Input: part model. Units: mm. Frame: model coordinates. Face numbers are marked on the shaded views. Give positions to 0.01 mm unless a question says otherwise; leave off trailing zeros. Loops run counter-clockwise (first coordinate to the right, second up) from the corner with the lowest first, then second, coordinate; pieces in that order, holes last. Notation, with made-up numbers: M 45,6.5 L 93,6.5 A23 cw 93,29.5 Z; hole C 50,15.25 d2. An arc over 180 degrees is marked long. Return JSON: item names as keys, results as strings. Group by question number.
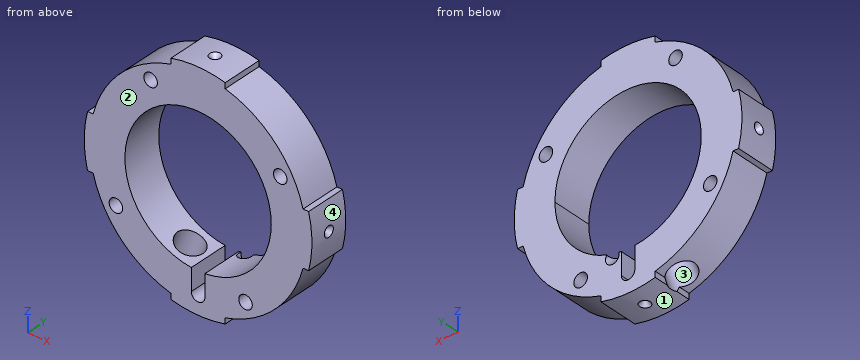
```python
from build123d import *

# Parameters (mm, degrees)
SKETCH1_R               = 40
BOSS_EXTRUDE1_DEPTH     = 15
BOSS_EXTRUDE2_DEPTH     = 15
CIRPATTERN1_COUNT       = 4
CUT_EXTRUDE1_REACH      = 102.194
CUT_EXTRUDE1_END_RADIUS = 27
SKETCH3_R               = 5
CUT_EXTRUDE2_REACH      = 63.262
SKETCH7_R               = 2.5
CIRPATTERN2_COUNT       = 4


with BuildPart() as part:
    # Sketch1 → Boss-Extrude1 (new body)
    with BuildSketch(Plane(origin=(0, 0, 0), x_dir=(1, 0, 0), z_dir=(0, 1, 0))):
        with Locations(Location((0, 0, 0), (0, 0, 270))):
            Circle(SKETCH1_R)
        with BuildLine():
            Line((-2.5, 26.884010118), (-2.5, 35))
            ThreePointArc((-2.5, 35), (0, 37.5), (2.5, 35))
            Line((2.5, 35), (2.5, 26.884010118))
            ThreePointArc((2.5, 26.884010118), (19.956202043, 18.186533479), (27, 0))
            ThreePointArc((27, 0), (-18.186533479, -19.956202043), (-2.5, 26.884010118))
        make_face(mode=Mode.SUBTRACT)
    extrude(amount=BOSS_EXTRUDE1_DEPTH)

    # Sketch2 → Boss-Extrude2 (add)
    with BuildSketch(Plane(origin=(0, 0, 0), x_dir=(1, 0, 0), z_dir=(0, 1, 0))):
        with BuildLine():
            Line((-10, 38.729833462), (-10, 40.792156109))
            ThreePointArc((-10, 40.792156109), (0, 42), (10, 40.792156109))
            Line((10, 40.792156109), (10, 38.729833462))
            ThreePointArc((10, 38.729833462), (0, 40), (-10, 38.729833462))
        make_face()
    boss_extrude2 = extrude(amount=BOSS_EXTRUDE2_DEPTH)

    # CirPattern1: Boss-Extrude2 ×4 about axis
    cirpattern1_axis = Axis((0, 0, 0), (0, 1, 0))
    for i in range(1, CIRPATTERN1_COUNT):
        add(boss_extrude2.rotate(cirpattern1_axis, i * 360 / CIRPATTERN1_COUNT))

    # Cut-Extrude1: up to this cylinder (the profile starts outside it)
    cut_extrude1_end = Plane(origin=(0, 7.5, 0), z_dir=(0, -1, 0)) * Cylinder(CUT_EXTRUDE1_END_RADIUS, 259.388, mode=Mode.PRIVATE)
    # Sketch3 → Cut-Extrude1 (cut, up to the surface)
    with BuildSketch(Plane(origin=(-14.36484602, 0, -39.467090073), x_dir=(0, -1, 0), z_dir=(-0.34202014332566616, 0, -0.9396926207859094)), mode=Mode.PRIVATE) as cut_extrude1_sk1:
        with Locations(Location((-7.5, 0, 0), (0, 0, 90))):
            Circle(SKETCH3_R)
    cut_extrude1_tool1 = extrude(cut_extrude1_sk1.sketch, amount=-CUT_EXTRUDE1_REACH, mode=Mode.PRIVATE) - cut_extrude1_end
    add(cut_extrude1_tool1.solids().sort_by_distance((-14.364846, 7.5, -39.46709))[0], mode=Mode.SUBTRACT)

    # Cut-Loft1: read off the stored shape, not the designer's step
    # Cut-Loft1: loft between two sections, ruled curve by curve
    cut_loft1_from = [
        Edge.make_bspline([(3.514240275, 15, -26.425622361), (3.43403107, 15, -26.617896283), (3.366678926, 15, -26.845149984), (3.307378731, 15, -27.375176333), (3.316276229, 15, -27.679385236), (3.439149004, 15, -28.164052423), (3.499144635, 15, -28.33030076), (3.660731431, 15, -28.657904123), (3.762322597, 15, -28.819259148), (4.01061992, 15, -29.122797357), (4.156634299, 15, -29.264354751), (4.484735709, 15, -29.510646827), (4.666742961, 15, -29.615210684), (5.051290806, 15, -29.775629094), (5.253649364, 15, -29.831407709), (5.659510988, 15, -29.891296475), (5.862836528, 15, -29.895470114), (6.253234588, 15, -29.858370786), (6.439375692, 15, -29.817046477), (6.785871072, 15, -29.701395244), (6.946225348, 15, -29.627068321), (7.37710147, 15, -29.373403645), (7.599547955, 15, -29.165702458), (7.934492045, 15, -28.750664024), (8.048605206, 15, -28.542917202), (8.209023616, 15, -28.158369358), (8.27637576, 15, -27.931115657), (8.335675954, 15, -27.401089308), (8.326778456, 15, -27.096880405), (8.203905682, 15, -26.612213219), (8.143910051, 15, -26.445964881), (7.982323255, 15, -26.118361518), (7.880732089, 15, -25.957006493), (7.632434766, 15, -25.653468284), (7.486420387, 15, -25.51191089), (7.158318977, 15, -25.265618814), (6.976311725, 15, -25.161054957), (6.59176388, 15, -25.000636547), (6.389405322, 15, -24.944857932), (5.983543698, 15, -24.884969166), (5.780218158, 15, -24.880795527), (5.389820098, 15, -24.917894855), (5.203678994, 15, -24.959219164), (4.857183614, 15, -25.074870397), (4.696829338, 15, -25.14919732), (4.265953216, 15, -25.402861996), (4.043506731, 15, -25.610563184), (3.708562641, 15, -26.025601617), (3.59444948, 15, -26.233348439), (3.514240275, 15, -26.425622361)], [0, 0, 0, 0, 0.0625, 0.0625, 0.125, 0.125, 0.15625, 0.15625, 0.1875, 0.1875, 0.21875, 0.21875, 0.25, 0.25, 0.28125, 0.28125, 0.3125, 0.3125, 0.34375, 0.34375, 0.375, 0.375, 0.4375, 0.4375, 0.5, 0.5, 0.5625, 0.5625, 0.625, 0.625, 0.65625, 0.65625, 0.6875, 0.6875, 0.71875, 0.71875, 0.75, 0.75, 0.78125, 0.78125, 0.8125, 0.8125, 0.84375, 0.84375, 0.875, 0.875, 0.9375, 0.9375, 1, 1, 1, 1], 3),
    ]
    cut_loft1_to = [
        Edge.make_bspline([(2.074985381, 12, -24.185039409), (2.13411013, 12, -24.427947342), (2.230529651, 12, -24.695535226), (2.549951041, 12, -25.250125143), (2.77479132, 12, -25.537914734), (3.238098263, 12, -25.919158327), (3.413256539, 12, -26.037240227), (3.802322838, 12, -26.239189581), (4.016282358, 12, -26.322904324), (4.47210154, 12, -26.439875089), (4.713892566, 12, -26.472945015), (5.206175894, 12, -26.477842878), (5.456469637, 12, -26.449562366), (5.942285504, 12, -26.331312867), (6.177577655, 12, -26.241399857), (6.612541462, 12, -26.010806383), (6.812086613, 12, -25.870313491), (7.163158835, 12, -25.556942174), (7.314710473, 12, -25.384260574), (7.567442578, 12, -25.026094956), (7.668738965, 12, -24.840722901), (7.90500687, 12, -24.28920003), (7.972433417, 12, -23.93027154), (8.001244839, 12, -23.290920383), (7.963900528, 12, -23.00895336), (7.845651029, 12, -22.523137493), (7.749231508, 12, -22.255549609), (7.429810118, 12, -21.700959692), (7.204969839, 12, -21.413170101), (6.741662897, 12, -21.031926508), (6.56650462, 12, -20.913844608), (6.177438321, 12, -20.711895254), (5.963478802, 12, -20.628180512), (5.507659619, 12, -20.511209746), (5.265868593, 12, -20.47813982), (4.773585266, 12, -20.473241957), (4.523291522, 12, -20.50152247), (4.037475655, 12, -20.619771968), (3.802183505, 12, -20.709684978), (3.367219697, 12, -20.940278452), (3.167674546, 12, -21.080771344), (2.816602324, 12, -21.394142661), (2.665050687, 12, -21.566824261), (2.412318581, 12, -21.924989879), (2.311022194, 12, -22.110361934), (2.074754289, 12, -22.661884805), (2.007327743, 12, -23.020813295), (1.97851632, 12, -23.660164452), (2.015860632, 12, -23.942131475), (2.074985381, 12, -24.185039409)], [0, 0, 0, 0, 0.0625, 0.0625, 0.125, 0.125, 0.15625, 0.15625, 0.1875, 0.1875, 0.21875, 0.21875, 0.25, 0.25, 0.28125, 0.28125, 0.3125, 0.3125, 0.34375, 0.34375, 0.375, 0.375, 0.4375, 0.4375, 0.5, 0.5, 0.5625, 0.5625, 0.625, 0.625, 0.65625, 0.65625, 0.6875, 0.6875, 0.71875, 0.71875, 0.75, 0.75, 0.78125, 0.78125, 0.8125, 0.8125, 0.84375, 0.84375, 0.875, 0.875, 0.9375, 0.9375, 1, 1, 1, 1], 3),
    ]
    cut_loft1 = Solid(Shell([*[Face.make_surface_from_curves(cut_loft1_from[k], cut_loft1_to[k]) for k in range(1)], Face(Wire(cut_loft1_from)), Face(Wire(cut_loft1_to))]))
    add(cut_loft1, mode=Mode.SUBTRACT)

    # Sketch7 → Cut-Extrude2 (cut, up to next)
    with BuildSketch(Plane(origin=(0, 15, 0), x_dir=(1, 0, 0), z_dir=(0, 1, 0)), mode=Mode.PRIVATE) as cut_extrude2_sk1:
        with Locations(Location((17.5, 30.310889132, 0), (0, 0, 270))):
            Circle(SKETCH7_R)
    cut_extrude2_tool1 = extrude(cut_extrude2_sk1.sketch, amount=-CUT_EXTRUDE2_REACH, mode=Mode.PRIVATE) & part.part
    # Sketch7 → Cut-Extrude2 (cut, up to next)
    with BuildSketch(Plane(origin=(0, 15, 0), x_dir=(1, 0, 0), z_dir=(0, 1, 0)), mode=Mode.PRIVATE) as cut_extrude2_sk2:
        with Locations(Location((30.310889132, -17.5, 0), (0, 0, 270))):
            Circle(SKETCH7_R)
    cut_extrude2_tool2 = extrude(cut_extrude2_sk2.sketch, amount=-CUT_EXTRUDE2_REACH, mode=Mode.PRIVATE) & part.part
    # Sketch7 → Cut-Extrude2 (cut, up to next)
    with BuildSketch(Plane(origin=(0, 15, 0), x_dir=(1, 0, 0), z_dir=(0, 1, 0)), mode=Mode.PRIVATE) as cut_extrude2_sk3:
        with Locations(Location((-17.5, -30.310889132, 0), (0, 0, 270))):
            Circle(SKETCH7_R)
    cut_extrude2_tool3 = extrude(cut_extrude2_sk3.sketch, amount=-CUT_EXTRUDE2_REACH, mode=Mode.PRIVATE) & part.part
    # Sketch7 → Cut-Extrude2 (cut, up to next)
    with BuildSketch(Plane(origin=(0, 15, 0), x_dir=(1, 0, 0), z_dir=(0, 1, 0)), mode=Mode.PRIVATE) as cut_extrude2_sk4:
        with Locations(Location((-30.310889132, 17.5, 0), (0, 0, 270))):
            Circle(SKETCH7_R)
    cut_extrude2_tool4 = extrude(cut_extrude2_sk4.sketch, amount=-CUT_EXTRUDE2_REACH, mode=Mode.PRIVATE) & part.part
    add(cut_extrude2_tool1.solids().sort_by_distance((17.5, 15, -30.310889))[0], mode=Mode.SUBTRACT)
    add(cut_extrude2_tool2.solids().sort_by_distance((30.310889, 15, 17.5))[0], mode=Mode.SUBTRACT)
    add(cut_extrude2_tool3.solids().sort_by_distance((-17.5, 15, 30.310889))[0], mode=Mode.SUBTRACT)
    add(cut_extrude2_tool4.solids().sort_by_distance((-30.310889, 15, -17.5))[0], mode=Mode.SUBTRACT)

    # Sketch9 → Cut-Revolve4 (revolve, cut)
    with BuildSketch(Plane(origin=(0, 0, 0), x_dir=(0, 0, -1), z_dir=(1, 0, 0)), mode=Mode.PRIVATE) as cut_revolve4_sk:
        Polygon((42, 7.5), (42, 5.5), (40, 7.5), align=None)
    cut_revolve4 = revolve(cut_revolve4_sk.sketch.rotate(Axis((0, 7.5, -40), (0, 0, -1)), 180), axis=Axis((0, 7.5, -40), (0, 0, -1)), mode=Mode.SUBTRACT)

    # CirPattern2: Cut-Revolve4 ×4 about axis
    cirpattern2_axis = Axis((0, 15, 0), (0, -1, 0))
    for i in range(1, CIRPATTERN2_COUNT):
        add(cut_revolve4.rotate(cirpattern2_axis, i * 360 / CIRPATTERN2_COUNT), mode=Mode.SUBTRACT)


solid = part.part
```
Item 1: Section B-B, the plane z = 4. Return loops of the section in (x, y), then the cut area to 3 significant figures.
Item 2: Section C-C, the plane z = 17. Return loops of the section in (x, y).
Item 3: Pull-direction query (X, two-part tool) for the marked faces 1, 2, 3 and 4; classes: pulls with the +X half, pulls with the -X half, needs draft (parallel to the pull), parting line crosses it, or undercut.
Item 4: Material intervals for line 1 (X direction, y = 7.5, z = -17.5); line 2 (X direction, y = 4.75, z = 15.5); line 3 (X direction, y = 10.25, z = 0), sorted ascending. Write a range as from..to.
Item 5: First-contact query: pin 1 Ø0.6 at (x, y) = (-39.5, 7) entering from -Z; pin 2 Ø2 at (x, y) = (14, 3.5) entering from -Z; pin 3 Ø1 at (y, z) = (13, -39.5) entering from -X; pin 4 Ø6 at (x, z) = (-27, 32.5) entering from -Y. Flat tips, straight axial feed; report the tip coordinate or a pass-through.
Item 6: Section A-A, the plane z = -17.5. Return loops of the section in (x, y), then the cut area to 3 significant figures.
Answer below:
{
 "1": {"outline": "M -41.81,0 L -26.7,0 L -26.7,15 L -41.81,15 Z; M 26.7,0 L 41.81,0 L 41.81,15 L 26.7,15 Z", "area": "453 mm^2"},
 "2": {"outline": "M -36.21,0 L -20.98,0 L -20.98,15 L -36.21,15 Z; M 20.98,0 L 27.86,0 L 27.86,15 L 20.98,15 Z; M 32.76,0 L 36.21,0 L 36.21,15 L 32.76,15 Z"},
 "3": {"face 1": "parting line crosses it", "face 2": "needs draft", "face 3": "undercut", "face 4": "pulls with the +X half"},
 "4": {"line 1": "-35.97..-32.81, -27.81..-20.56, 20.56..35.97", "line 2": "-36.87..-22.11, 22.11..28.81, 31.81..36.87", "line 3": "-42..-27, 27..42"},
 "5": {"pin 1": "z = -10", "pin 2": "z = -37.83", "pin 3": "x = -10", "pin 4": "y = 0"},
 "6": {"outline": "M -35.97,0 L -32.81,0 L -32.81,15 L -35.97,15 Z; M -27.81,0 L -20.56,0 L -20.56,15 L -27.81,15 Z; M 20.56,0 L 35.97,0 L 35.97,15 L 20.56,15 Z", "area": "387 mm^2"}
}
